from build123d import *

# Parameters (mm, degrees)
F0_W     = 80
F0_H     = 100
F1_DEPTH = 5
F2_W     = 120
F2_H     = 10
F3_DEPTH = 120
F5_DEPTH = 25
F6_R     = 6
F7_DEPTH = 25


with BuildPart() as f1:
    # F0 (on Front) → F1 (new body, symmetric)
    with BuildSketch(Plane.XZ):
        Rectangle(F0_W, F0_H)
    extrude(amount=F1_DEPTH, both=True)

    # F2 (on face) → F3 (join)
    with BuildSketch(Plane.XZ.offset(5)):
        with Locations((-20, -45)):
            Rectangle(F2_W, F2_H)
    extrude(amount=-F3_DEPTH)

    # F4 (on face) → F5 (cut)
    with BuildSketch(Plane.XY.offset(-40)):
        with BuildLine():
            ThreePointArc((20, 79), (18.242641, 83.242641), (14, 85))
            Line((14, 85), (-54, 85))
            ThreePointArc((-54, 85), (-58.242641, 83.242641), (-60, 79))
            ThreePointArc((-60, 79), (-58.242641, 74.757359), (-54, 73))
            Line((-54, 73), (14, 73))
            ThreePointArc((14, 73), (18.242641, 74.757359), (20, 79))
        make_face()
        with BuildLine():
            Line((-54, 28), (14, 28))
            ThreePointArc((14, 28), (18.242641, 29.757359), (20, 34))
            ThreePointArc((20, 34), (18.242641, 38.242641), (14, 40))
            Line((14, 40), (-54, 40))
            ThreePointArc((-54, 40), (-58.242641, 38.242641), (-60, 34))
            ThreePointArc((-60, 34), (-58.242641, 29.757359), (-54, 28))
        make_face()
    extrude(amount=-F5_DEPTH, mode=Mode.SUBTRACT)

    # F6 (on face) → F7 (cut)
    with BuildSketch(Plane(origin=(0, 5, 0), x_dir=(-1, 0, 0), z_dir=(0, 1, 0))):
        with Locations((-15, 25)):
            Circle(F6_R)
        with Locations((15, -10)):
            Circle(F6_R)
    extrude(amount=-F7_DEPTH, mode=Mode.SUBTRACT)


solid = f1.part
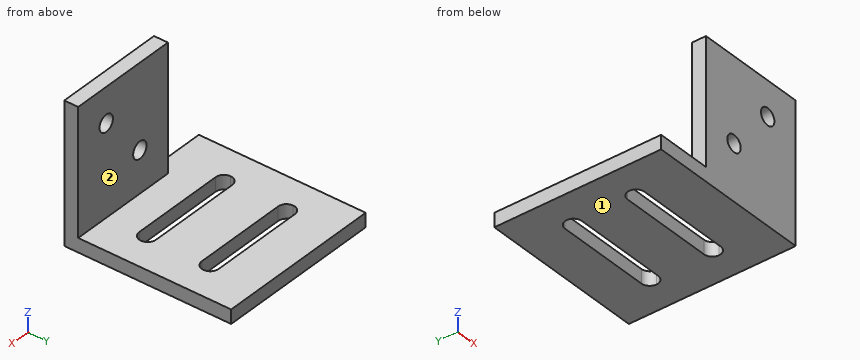
Design review of the part built by this model. Coordinates are the model's own, in mm. Face numbers are marked on the shaded views. A direction names the side the tool comes from. Give positions to 0.01 mm unless a question says otherwise; leave off trailing zeros. Loops run counter-clockwise (first coordinate to the right, second up) from the corner with the lowest first, then second, coordinate; pieces in that order, holes last. Notation, with made-up numbers: M 4,24 L 11,24 A17 ccw 11,47 Z; hole C -20,-33 d2. An arc over 180 degrees is marked long. Write item = value, one per line.
Q1. Insertion check: pin 1 (9.5 mm diameter, centred on x = 15, z = 25, fed in from +Y); pin 2 (3 mm diameter, centred on y = 1, z = 14, fed in from -X); pin 3 (5 mm diameter, centred on x = -14.5, z = 20.5, fed in from +Y); pin 4 (8 mm diameter, centred on x = -18, y = 96.5, fed in from +Z). Each pin has a flat end and moves straight along its axis. Give the tip position at first contact, or say it passes through.
Output values:
pin_1 = through
pin_2 = -40
pin_3 = 5
pin_4 = -40
Q2. To check wall thickness, follow line 1 (Z direction, x = 15, y = -2); line 2 (Z direction, x = -63, y = 17.5); line 3 (Y direction, x = 6, z = -5). State the ranges of each line that lie inside material, in increasing order. Write a range as [from, to].
Output values:
line_1 = [-50, 19], [31, 50]
line_2 = [-50, -40]
line_3 = [-5, 5]
Q3. We need section D-D (x = 23.5). Give the boundary of the cut face in (y, z), plus the area to 3 significant figures.
Output values:
outline = M -5,-50 L 115,-50 L 115,-40 L 5,-40 L 5,50 L -5,50 Z
area = 2,100 mm^2
Q4. We need section C-C (y = 81.5). Give the boundary of the cut face in (x, z).
Output values:
outline = M -80,-50 L -59.45,-50 L -59.45,-40 L -80,-40 Z; M 19.45,-50 L 40,-50 L 40,-40 L 19.45,-40 Z
Q5. We need section B-B (z = 25). Give the boundary of the cut face in (x, y).
Output values:
outline = M -40,-5 L 9,-5 L 9,5 L -40,5 Z; M 21,-5 L 40,-5 L 40,5 L 21,5 Z
Q6. For the marked faces 1 and 2, list the 3-axis set-ups (+Z, -Z, +X, -X, +Y, -Y) from which the entire face can be reached by the end or side of a thin tool; tool diameter is ignored.
Output values:
face_1 = -Z, +X, -X, +Y, -Y
face_2 = +Z, +X, -X, +Y
Q7. We need section A-A (x = -15). Give the boundary of the cut face in (y, z).
Output values:
outline = M -5,-50 L 28,-50 L 28,-40 L 5,-40 L 5,-16 L -5,-16 Z; M -5,-4 L 5,-4 L 5,50 L -5,50 Z; M 40,-50 L 73,-50 L 73,-40 L 40,-40 Z; M 85,-50 L 115,-50 L 115,-40 L 85,-40 Z
